```python
from build123d import *

# Parameters (mm, degrees)
SKETCH1_W           = 86
SKETCH1_H           = 50
BOSS_EXTRUDE2_DEPTH = 6
BOSS_EXTRUDE3_DEPTH = 50
SKETCH4_R           = 8
CUT_EXTRUDE1_DEPTH  = 121
BOSS_EXTRUDE5_DEPTH = 50
BOSS_EXTRUDE6_DEPTH = 50
FILLET1_R           = 5
FILLET2_R           = 5
FILLET3_R           = 5
FILLET4_R           = 5
FILLET5_R           = 5
SKETCH7_R           = 1.5
CUT_EXTRUDE2_DEPTH  = 50
SKETCH8_R           = 1.5
CUT_EXTRUDE4_DEPTH  = 50
SKETCH9_W           = 76
SKETCH9_H           = 50
BOSS_EXTRUDE7_DEPTH = 5
CUT_EXTRUDE5_DEPTH  = 121


with BuildPart() as part:
    # Sketch1 → Boss-Extrude2 (new body)
    with BuildSketch(Plane.XY):
        with Locations((43, 25)):
            Rectangle(SKETCH1_W, SKETCH1_H)
    extrude(amount=BOSS_EXTRUDE2_DEPTH)

    # Sketch2 → Boss-Extrude3 (add)
    with BuildSketch(Plane(origin=(0, 0, 0), x_dir=(-1, 0, 0), z_dir=(0, -1, 0))):
        with BuildLine():
            Line((-61, -21), (-61, -6))
            Line((-61, -6), (-25, -6))
            Line((-25, -6), (-25, -21))
            ThreePointArc((-25, -21), (-43, -39), (-61, -21))
        make_face()
    extrude(amount=-BOSS_EXTRUDE3_DEPTH)

    # Sketch4 → Cut-Extrude1 (cut)
    with BuildSketch(Plane(origin=(0, 0, 0), x_dir=(-1, 0, 0), z_dir=(0, -1, 0))):
        with Locations(Location((-43, -21, 0), (0, 0, 90))):
            Circle(SKETCH4_R)
    extrude(amount=-CUT_EXTRUDE1_DEPTH, mode=Mode.SUBTRACT)

    # Sketch5 → Boss-Extrude5 (add)
    with BuildSketch(Plane(origin=(0, 0, 0), x_dir=(-1, 0, 0), z_dir=(0, -1, 0))):
        Polygon((-61, -6), (-73.5, -6), (-61, -18.5), align=None)
    extrude(amount=-BOSS_EXTRUDE5_DEPTH)

    # Sketch6 → Boss-Extrude6 (add)
    with BuildSketch(Plane(origin=(0, 0, 0), x_dir=(-1, 0, 0), z_dir=(0, -1, 0))):
        Polygon((-25, -6), (-12.5, -6), (-25, -18.5), align=None)
    extrude(amount=-BOSS_EXTRUDE6_DEPTH)

    # Fillet1
    fillet1_edges = [part.edges().sort_by_distance(p)[0] for p in [
        (86, 25, 6),
    ]]
    fillet(fillet1_edges, radius=FILLET1_R)

    # Fillet2
    fillet2_edges = [part.edges().sort_by_distance(p)[0] for p in [
        (73.5, 25, 6),
    ]]
    fillet(fillet2_edges, radius=FILLET2_R)

    # Fillet3
    fillet3_edges = [part.edges().sort_by_distance(p)[0] for p in [
        (61, 25, 18.5),
    ]]
    fillet(fillet3_edges, radius=FILLET3_R)

    # Fillet4
    fillet4_edges = [part.edges().sort_by_distance(p)[0] for p in [
        (25, 25, 18.5),
        (0, 25, 6),
        (12.5, 25, 6),
    ]]
    fillet(fillet4_edges, radius=FILLET4_R)

    # Fillet5
    fillet5_edges = [part.edges().sort_by_distance(p)[0] for p in [
        (43, 0, 39),
        (61, 0, 20.785533906),
        (43, 50, 39),
        (61, 50, 20.785533906),
        (78.285533906, 50, 6),
        (86, 50, 0.5),
        (84.535533906, 50, 4.535533906),
        (86, 0, 0.5),
        (84.535533906, 0, 4.535533906),
        (78.285533906, 0, 6),
        (67.25, 0, 12.25),
        (67.25, 50, 12.25),
        (73.65765065, 0, 6.380602337),
        (73.65765065, 50, 6.380602337),
        (61.380602337, 0, 18.65765065),
        (61.380602337, 50, 18.65765065),
        (18.75, 0, 12.25),
        (18.75, 50, 12.25),
        (7.714466094, 50, 6),
        (7.714466094, 0, 6),
        (25, 50, 20.785533906),
        (25, 0, 20.785533906),
        (0, 0, 0.5),
        (1.464466094, 0, 4.535533906),
        (0, 50, 0.5),
        (1.464466094, 50, 4.535533906),
        (12.34234935, 0, 6.380602337),
        (12.34234935, 50, 6.380602337),
        (24.619397663, 0, 18.65765065),
        (24.619397663, 50, 18.65765065),
    ]]
    fillet(fillet5_edges, radius=FILLET5_R)

    # Sketch7 → Cut-Extrude2 (cut)
    with BuildSketch(Plane.XY.offset(6)):
        with Locations((7.714466094, 35.601677871)):
            Circle(SKETCH7_R)
        with Locations((7.714466094, 14.398322129)):
            Circle(SKETCH7_R)
    extrude(amount=-CUT_EXTRUDE2_DEPTH, mode=Mode.SUBTRACT)

    # Sketch8 → Cut-Extrude4 (cut)
    with BuildSketch(Plane.XY.offset(6)):
        with Locations((78.285533906, 35.60168)):
            Circle(SKETCH8_R)
        with Locations((78.285533906, 14.39832)):
            Circle(SKETCH8_R)
    extrude(amount=-CUT_EXTRUDE4_DEPTH, mode=Mode.SUBTRACT)

    # Sketch9 → Boss-Extrude7 (add)
    with BuildSketch(Plane(origin=(0, 0, 0), x_dir=(-1, 0, 0), z_dir=(0, 0, -1))):
        with Locations((-43, 25)):
            Rectangle(SKETCH9_W, SKETCH9_H)
    extrude(amount=BOSS_EXTRUDE7_DEPTH)

    # Sketch11 → Cut-Extrude5 (cut)
    with BuildSketch(Plane.ZY.offset(-5)):
        Polygon((0, 50), (-2.260657521, -1.777569844), (-5.022686567, -1.777569844), (-5, 50), align=None)
    extrude(amount=-CUT_EXTRUDE5_DEPTH, mode=Mode.SUBTRACT)


solid = part.part
```
Work out the finished part from the listing and answer in its coordinate system (mm). A direction names the side the tool comes from. Coordinates: 2 decimals unless noted, no trailing zeros. Loops run counter-clockwise (first coordinate to the right, second up) from the corner with the lowest first, then second, coordinate; pieces in that order, holes last.
1) Flat-ended cylindrical pins translate along their axes: pin 1 (1.5 mm diameter, centred on y = 23.5, z = 12.5, fed in from +X); pin 2 (6 mm diameter, centred on x = 7.5, y = 18, fed in from +Z); pin 3 (1.8 mm diameter, centred on x = 7.71, y = 14.4, fed in from +Z). Find the tip coordinate at first contact, or state that the pin passes through.
Results:
pin 1: stops at x = 67.75
pin 2: stops at z = 6
pin 3: stops at z = 0
2) Section B-B (y = 7.5) is taken. Give the vertices of the cut face in (x, z), plus the area to 3 significant figures.
Results:
outline: (0, 0) - (5, 0) - (5, -1.86) - (81, -1.86) - (81, 0) - (86, 0) - (86, 1) arc R5 ccw to (81, 6) - (75.57, 6) arc R5 cw to (72.04, 7.46) - (62.46, 17.04) arc R5 cw to (61, 20.57) - (61, 21) arc R18 ccw to (25, 21) - (25, 20.57) arc R5 cw to (23.54, 17.04) - (13.96, 7.46) arc R5 cw to (10.43, 6) - (5, 6) arc R5 ccw to (0, 1) - close; hole circle Ø16 at (43, 21)
area: 1,650 mm2
3) Section C-C (y = 44) is taken. Give the vertices of the cut face in (x, z), plus the area to 3 significant figures.
Results:
outline: (0, 0) - (5, 0) - (5, -0.26) - (81, -0.26) - (81, 0) - (86, 0) - (86, 1) arc R5 ccw to (81, 6) - (75.57, 6) arc R5 cw to (72.04, 7.46) - (62.46, 17.04) arc R5 cw to (61, 20.57) - (61, 21) arc R18 ccw to (25, 21) - (25, 20.57) arc R5 cw to (23.54, 17.04) - (13.96, 7.46) arc R5 cw to (10.43, 6) - (5, 6) arc R5 ccw to (0, 1) - close; hole circle Ø16 at (43, 21)
area: 1,530 mm2
4) For faces 5 (the cylindrical face through (8, 48, 5)), 6 (the flat face through (5, 19, -1)), 7 (the cylindrical face through (76.787, 14.464, 3.042)), determine the directions among +Z, -Z, +X, -X, +Y, -Y from which every point of the face is accessible in a straight line to the end or side of a thin tool.
Results:
face 5: +Z, -X, +Y
face 6: -Z, -X, +Y, -Y
face 7: +Z
5) Consider probe 1 along Z at (x, y) = (40.5, 41.5); probe 2 along X at (y, z) = (45.5, 18); probe 3 along Y at (x, z) = (30, 30). Determine where each line is inside the solid, lowest interval first.
Results:
probe 1: z = -0.37 to 13.4, 28.6 to 38.83
probe 2: x = 24.32 to 35.58, 50.42 to 61.68
probe 3: y = 0.87 to 49.13
6) For a pull along X with two mould halves and no side action, classify faces 1 (the cylindrical face through (19.83, 48.5, 11.31)), 2 (the cylindrical face through (7.389, 34.137, 3.042)), 3 (the cylindrical face through (84.57, 48.5, 0.49)), 4 (the flat face through (78, 14, 0)) as +X half, -X half, draft (parallel to the pull), parting line (faces both ways), or undercut.
Results:
face 1: -X half
face 2: undercut
face 3: +X half
face 4: undercut
7) Section A-A (x = 43) is taken. Give the vertices of the cut face in (y, z).
Results:
outline: (0, -2.18) - (50, 0) - (50, 13) - (0, 13) - close; (0, 29) - (50, 29) - (50, 34) arc R5 ccw to (45, 39) - (5, 39) arc R5 ccw to (0, 34) - close
